Read the model definition and answer for the solid it produces. Units are mm, in the model's axes. Face numbers are marked on the shaded views. A direction names the side the tool comes from. Give positions to 0.01 mm unless a question says otherwise; leave off trailing zeros. Write each loop counter-clockwise with the first axis right and the second up, starting at its lowest first coordinate (ties: lowest second). Pieces come first, ordered by that corner, then holes. Notation, with made-up numbers: (-12.5, -21.75) -> (14.5, -21.75) arc R16 cw to (14.5, -7.75) -> close; hole circle Ø11 at (-3, 32). An arc over 180 degrees is marked (long way). Write item = value, one per line.
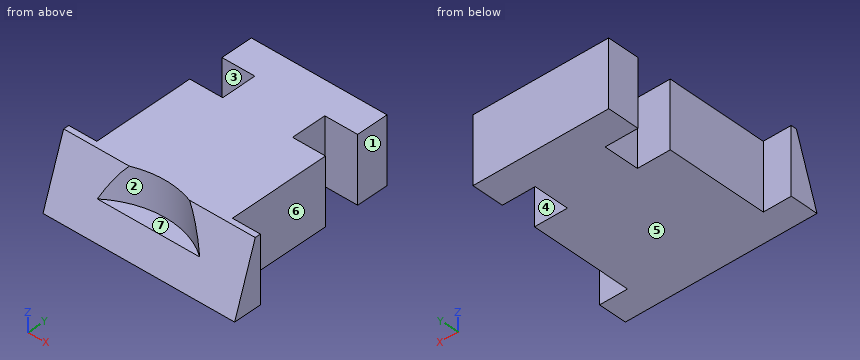
from build123d import *

# Parameters (mm, degrees)
SKETCH1_W           = 12.319
SKETCH1_H           = 6
BOSS_EXTRUDE1_DEPTH = 15.24
SKETCH1_3_W         = 12.319
SKETCH1_3_H         = 6
SKETCH1_3_W_2       = 2.54
BOSS_EXTRUDE2_DEPTH = 2.54
SKETCH2_W           = 2.9845
SKETCH2_H           = 3.175
CUT_EXTRUDE1_DEPTH  = 19.545589779
CUT_EXTRUDE2_DEPTH  = 24.323438876
SKETCH4_R           = 7.62
CUT_EXTRUDE3_DEPTH  = 3.175


with BuildPart() as part:
    # Sketch1 → Boss-Extrude1 (new body)
    with BuildSketch(Plane(origin=(0, 0, 0), x_dir=(1, 0, 0), z_dir=(0, 1, 0))):
        Rectangle(SKETCH1_W, SKETCH1_H)
    extrude(amount=BOSS_EXTRUDE1_DEPTH)

    # Sketch1_3 → Boss-Extrude2 (add)
    with BuildSketch(Plane(origin=(0, 0, 0), x_dir=(1, 0, 0), z_dir=(0, 1, 0))):
        Rectangle(SKETCH1_3_W, SKETCH1_3_H)
        with Locations((7.4295, 0)):
            Rectangle(SKETCH1_3_W_2, SKETCH1_3_H)
        with Locations((-7.4295, 0)):
            Rectangle(SKETCH1_3_W_2, SKETCH1_3_H)
    extrude(amount=-BOSS_EXTRUDE2_DEPTH)

    # Sketch2 → Cut-Extrude1 (cut, through all)
    with BuildSketch(Plane(origin=(0, 0, -3), x_dir=(-1, 0, 0), z_dir=(0, 0, -1))):
        with Locations((-4.66725, 10.7625)):
            Rectangle(SKETCH2_W, SKETCH2_H)
        with Locations((4.66725, 10.7625)):
            Rectangle(SKETCH2_W, SKETCH2_H)
    extrude(amount=-CUT_EXTRUDE1_DEPTH, mode=Mode.SUBTRACT)

    # Sketch3 → Cut-Extrude2 (cut, through all)
    with BuildSketch(Plane.ZY.offset(8.6995)):
        Polygon((-3, -2.54), (3, -0.508), (3, -2.54), align=None)
    extrude(amount=-CUT_EXTRUDE2_DEPTH, mode=Mode.SUBTRACT)

    # Sketch4 → Cut-Extrude3 (cut)
    with BuildSketch(Plane.XY.offset(3)):
        with Locations((0, -7.62)):
            Circle(SKETCH4_R)
    extrude(amount=-CUT_EXTRUDE3_DEPTH, mode=Mode.SUBTRACT)


solid = part.part
(1) A tool of negligible diameter and unlimited length cuts with its end or side. For the marked faces 1, 2, 3 and 4, from which of +Z, -Z, +X, -X, +Y, -Y can it reach the whole face along a straight path? Write none if from no direction.
Checks:
face_1 = +Z, -Z, +X, +Y
face_2 = +Z, -Y
face_3 = +Z, -Z, -X
face_4 = +Z, -Z, +X
(2) The part is cut by section C-C on y = 6. Determine the outline of the cut face in (x, z).
Checks:
outline = (-6.16, -3) -> (6.16, -3) -> (6.16, 3) -> (-6.16, 3) -> close
(3) Consider L1, parallel to X at y = 13.25, z = -0.5; L2, parallel to Y at x = -5, z = 1.75 (3 decimals); L3, parallel to Y at x = -5, z = 2.5 (3 decimals). Determine where each line is inside the solid, lowest interval first.
Checks:
L1 = -6.16 to 6.16
L2 = -0.931 to 9.175, 12.35 to 15.24
L3 = -0.677 to 9.175, 12.35 to 15.24
(4) The part is cut by section A-A on x = -4.25. Determine the outline of the cut face in (y, z) (3 decimals), plus the area to 3 significant figures.
Checks:
outline = (-2.54, -3) -> (9.175, -3) -> (9.175, 3) -> (-0.508, 3) -> (-1.295, 0.675) -> (-1.295, -0.175) -> (-1.583, -0.175) -> close; (12.35, -3) -> (15.24, -3) -> (15.24, 3) -> (12.35, 3) -> close
area = 81.4 mm²
(5) For a pull along Z with two mould halves and no side action, classify the marked faces 5, 6 and 7 as released by +Z, released by -Z, zero draft, split by the parting line, or undercut.
Checks:
face_5 = released by -Z
face_6 = zero draft
face_7 = released by +Z
(6) Given P1, Ø3, axis at y = 6.5, z = 0, coming from the +X side; P2, Ø1.4, axis at y = 14, z = 1, coming from the -X side; P3, Ø1.5, axis at x = 5, y = 11, coming from the -Z side; P4, Ø0.9, axis at x = -5, z = -0.5, coming from the -Y side, each flat-ended and moving along its own axis, determine where each tip first touches the part or whether it passes through.
Checks:
P1 = 6.16
P2 = -6.16
P3 = through
P4 = -1.85
(7) The part is cut by section D-D on x = -1.5. Determine the outline of the cut face in (y, z) (3 decimals).
Checks:
outline = (-2.54, -3) -> (15.24, -3) -> (15.24, 3) -> (-0.149, 3) -> (-0.149, -0.175) -> (-1.583, -0.175) -> close
